Study the drawing (mm; zero at the part's minimum x, y, z) and answer. A direction names the side the tool comes from. Round coordinates to 2 decimals unless told otherwise and drop trailing zeros. Write each loop counter-clockwise with the first axis right and the second up, starting at its lowest first coordinate (ties: lowest second). Pieces come first, ordered by that corner, then holes.
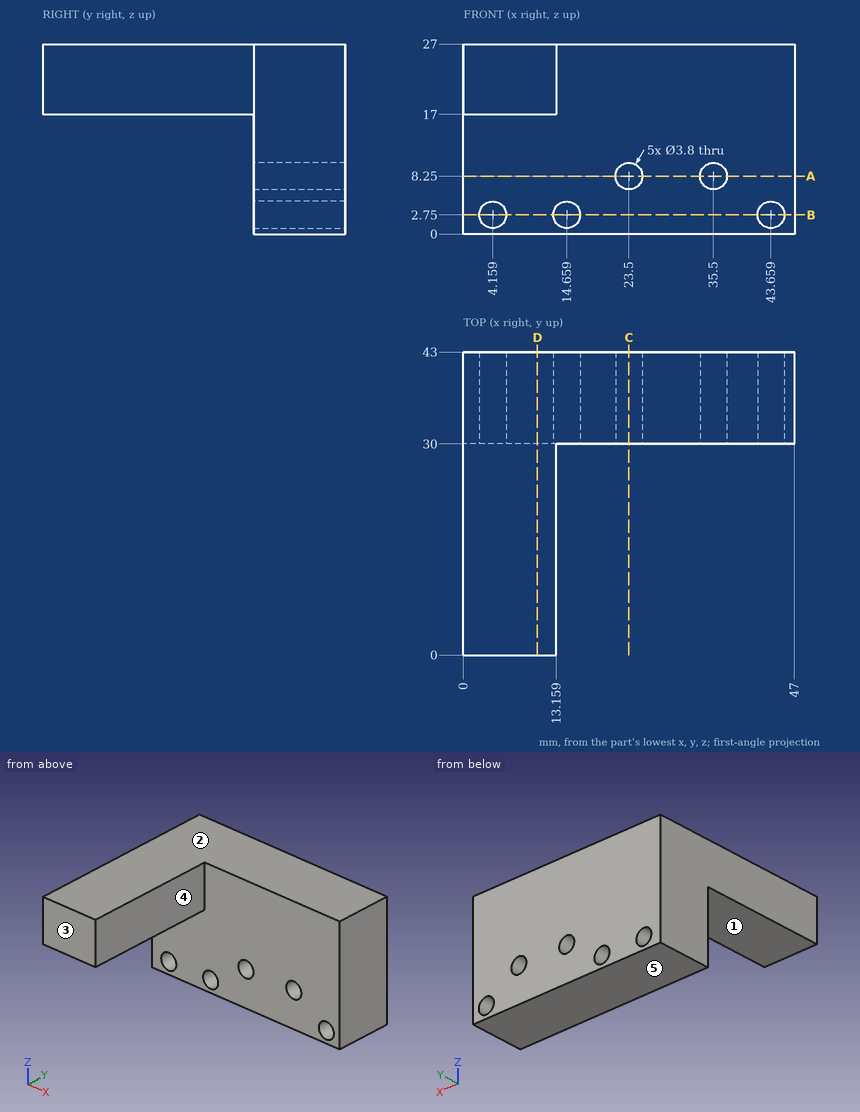
Q1. Find section A-A (z = 8.25). Determine the outline of the cut face in (x, y).
Q2. A tool of negligible diameter and unlimited length cuts with its end or side. For the marked faces 4 and 5, from which of +Z, -Z, +X, -X, +Y, -Y can it reach the whole face along a straight path? Write none if from no direction.
Q3. Find section C-C (x = 23.5). Determine the outline of the cut face in (y, z), plus the area to 3 significant figures.
Q4. Find section D-D (x = 10.5). Determine the outline of the cut face in (y, z), plus the area to 3 significant figures.
Q5. The mould has two halves that part along Z. Classify the marked faces 1, 2 and 3: +Z half, -Z half, draft (parallel to the pull), parting line (faces both ways), or undercut.
Q6. Find the intervals of material crossed by L1, parallel to X at y = 32.5, z = 8.25; L2, parallel to X at y = 39, z = 2.75; L3, parallel to Y at x = 40.5, z = 23.75, in increasing order.
Q7. Given pin 1 (3 mm diameter, centred on x = 14.66, z = 2.75, fed in from +Y); pin 2 (5 mm diameter, centred on x = 18, y = 31.5, fed in from -Z); pin 3 (1.5 mm diameter, centred on y = 19.5, z = 18.5, fed in from +X); pin 4 (8 mm diameter, centred on x = 19, z = 9, fed in from -Y), each flat-ended and moving along its own axis, determine where each tip first touches the part or whether it passes through.
Q8. Find section B-B (z = 2.75). Determine the outline of the cut face in (x, y).
Report:
1. outline: (0, 30) - (21.6, 30) - (21.6, 43) - (0, 43) - close; (25.4, 30) - (33.6, 30) - (33.6, 43) - (25.4, 43) - close; (37.4, 30) - (47, 30) - (47, 43) - (37.4, 43) - close
2. face 4: +Z, -Z, +X, -Y
2. face 5: -Z, +X, -X, +Y, -Y
3. outline: (30, 0) - (43, 0) - (43, 6.35) - (30, 6.35) - close; (30, 10.15) - (43, 10.15) - (43, 27) - (30, 27) - close
3. area: 302 mm2
4. outline: (0, 17) - (30, 17) - (30, 0) - (43, 0) - (43, 27) - (0, 27) - close
4. area: 651 mm2
5. face 1: -Z half
5. face 2: +Z half
5. face 3: draft
6. L1: x = 0 to 21.6, 25.4 to 33.6, 37.4 to 47
6. L2: x = 0 to 2.26, 6.06 to 12.76, 16.56 to 41.76, 45.56 to 47
6. L3: y = 30 to 43
7. pin 1: passes through
7. pin 2: stops at z = 0
7. pin 3: stops at x = 13.16
7. pin 4: stops at y = 30
8. outline: (0, 30) - (2.26, 30) - (2.26, 43) - (0, 43) - close; (6.06, 30) - (12.76, 30) - (12.76, 43) - (6.06, 43) - close; (16.56, 30) - (41.76, 30) - (41.76, 43) - (16.56, 43) - close; (45.56, 30) - (47, 30) - (47, 43) - (45.56, 43) - close
